The listing builds one solid part. Answer for the finished solid, in the listing's coordinates (mm). A direction names the side the tool comes from. Give positions to 0.01 mm unless a question says otherwise; leave off trailing zeros. Loops run counter-clockwise (first coordinate to the right, second up) from the corner with the lowest first, then second, coordinate; pieces in that order, holes last. Notation, with made-up numbers: M 13,-16 L 23,-16 A11 ccw 23,-11 Z; hole C -5,24.25 d10. An arc over 180 degrees is marked long. One line per item, written item: value. Start each with the question number.
Q1. A cutting plane is placed at C-C, the plane z = -20.3. Determine the outline of the cut face in (x, y), and give its area (3 significant figures).
Q2. A cutting plane is placed at B-B, the plane x = 1.65. Determine the outline of the cut face in (y, z), and give its area (3 significant figures).
Q3. The mould has two halves that part along Y. Classify faces 3 (the cylindrical face through (-0.04, 8.54, -41.03)), 4 (the cylindrical face through (1, 9, -48)), 5 (the cylindrical face through (0.035, -3.212, -2.502)): +Y half, -Y half, draft (parallel to the pull), parting line (faces both ways), or undercut.
Q4. A cutting plane is placed at D-D, the plane z = -39.5. Determine the outline of the cut face in (x, y).
Q5. Consider L1, parallel to Y at x = -0.15, z = -20.3; L2, parallel to Y at x = -1.9, z = -29.5; L3, parallel to Y at x = -1.4, z = -40. Determine where each line is inside the solid, lowest interval first.
Q6. Flat-ended cylindrical pins translate along their axes: pin 1 (1.5 mm diameter, centred on x = 1, z = -28, fed in from +Y); pin 2 (3 mm diameter, centred on x = 1, y = -8, fed in from +Z). Find the tip coordinate at first contact, or state that the pin passes through.
Q7. For faces 1 (the flat face through (-2.5, -1, -25)), 2 (the flat face through (1, 10, -53)), determine the directions among +Z, -Z, +X, -X, +Y, -Y from which every point of the face is accessible in a straight line to the end or side of a thin tool.
Q8. A cutting plane is placed at A-A, the plane y = -10.8. Determine the outline of the cut face in (x, z), and give its area (3 significant figures).
from build123d import *

# Parameters (mm, degrees)
ESQUISSE1_W             = 5
ESQUISSE1_H             = 28
EXTRUSION1_DEPTH        = 46
ESQUISSE2_R             = 2
ESQUISSE2_R_2           = 3.5
EXTRUSION2_DEPTH        = 49.342527861
TROU_TARAUD_M21_D       = 1.6
BOSS_EXTRU_2_DEPTH      = 5
ENL_V_MAT_EXTRU_1_DEPTH = 10
ENL_V_START             = 3
ENL_V_MAT_EXTRU_2_DEPTH = 56.9067059


with BuildPart() as part:
    # Esquisse1 → Extrusion1 (new body)
    with BuildSketch(Plane.XY):
        Rectangle(ESQUISSE1_W, ESQUISSE1_H)
    extrude(amount=-EXTRUSION1_DEPTH)

    # Esquisse2 → Extrusion2 (cut, through all)
    with BuildSketch(Plane(origin=(2.5, 0, 0), x_dir=(0, 0, -1), z_dir=(1, 0, 0))):
        with Locations((4.5, -3.3)):
            Circle(ESQUISSE2_R)
        with Locations((40, -3.3)):
            Circle(ESQUISSE2_R_2)
    extrude(amount=-EXTRUSION2_DEPTH, mode=Mode.SUBTRACT)

    # Trou taraudé M21 (through all)
    with Locations(Plane(origin=(2.5, 0, 0), x_dir=(0, 0, -1), z_dir=(1, 0, 0))):
        with Locations((20.3, 4.2), (20.3, -10.8)):
            Hole(TROU_TARAUD_M21_D / 2)

    # Esquisse12 → Boss.-Extru.2 (add)
    with BuildSketch(Plane.ZY.offset(2.5)):
        with BuildLine():
            Line((-46, 14), (-50.208712153, 14))
            ThreePointArc((-50.208712153, 14), (-52.5, 12.5), (-54.791287847, 14))
            Line((-54.791287847, 14), (-55, 14))
            ThreePointArc((-55, 14), (-57, 12), (-55, 10))
            Line((-55, 10), (-50, 10))
            ThreePointArc((-50, 10), (-48.294604063, 9.328011132), (-47.506013794, 7.673299759))
            Line((-47.506013794, 7.673299759), (-46, -14))
            Line((-46, -14), (-46, 14))
        make_face()
    extrude(amount=-BOSS_EXTRU_2_DEPTH)

    # Esquisse13 → Enlèv. mat.-Extru.1 (cut)
    with BuildSketch(Plane.ZY.offset(2.5)):
        with BuildLine():
            ThreePointArc((-47.521517479, 7.82729863), (-47.512573575, 7.750419205), (-47.506013794, 7.673299759))
            Line((-47.506013794, 7.673299759), (-46, -14))
            Line((-46, -14), (-36, -14))
            ThreePointArc((-36, -14), (-37.164860583, -13.780452956), (-38.169882605, -13.151937389))
            Line((-38.169882605, -13.151937389), (-44.068529884, -7.709882605))
            ThreePointArc((-44.068529884, -7.709882605), (-45.326210473, -6.062513711), (-45.94835805, -4.085516713))
            Line((-45.94835805, -4.085516713), (-47.521517479, 7.82729863))
        make_face()
        with BuildLine():
            ThreePointArc((-18.401732057, -13.767179458), (-18.989661678, -13.941255662), (-19.6, -14))
            Line((-19.6, -14), (0, -14))
            Line((0, -14), (0, -3.3))
            ThreePointArc((0, -3.3), (-0.769531576, -5.81666552), (-2.814935705, -7.472596113))
            Line((-2.814935705, -7.472596113), (-18.401732057, -13.767179458))
        make_face()
        with BuildLine():
            ThreePointArc((-2.814935705, 0.872596113), (-0.769531576, -0.78333448), (0, -3.3))
            Line((0, -3.3), (0, 14))
            Line((0, 14), (-50, 14))
            ThreePointArc((-50, 14), (-47.228274994, 13.379416679), (-44.985807313, 11.636166305))
            ThreePointArc((-44.985807313, 11.636166305), (-40.96713796, 8.512131601), (-36, 7.4))
            Line((-36, 7.4), (-19.6, 7.4))
            ThreePointArc((-19.6, 7.4), (-18.989661678, 7.341255662), (-18.401732057, 7.167179458))
            Line((-18.401732057, 7.167179458), (-2.814935705, 0.872596113))
        make_face()
    extrude(amount=-ENL_V_MAT_EXTRU_1_DEPTH, mode=Mode.SUBTRACT)

    # Esquisse14 → Enlèv. mat.-Extru.2 (cut, through all)
    with BuildSketch(Plane.ZY.offset(-2.5).offset(ENL_V_START)):
        with BuildLine():
            ThreePointArc((-44.985807313, 11.636166305), (-47.228274994, 13.379416679), (-50, 14))
            Line((-50, 14), (-50.208712153, 14))
            ThreePointArc((-50.208712153, 14), (-52.5, 12.5), (-54.791287847, 14))
            Line((-54.791287847, 14), (-55, 14))
            ThreePointArc((-55, 14), (-57, 12), (-55, 10))
            Line((-55, 10), (-50, 10))
            ThreePointArc((-50, 10), (-48.933951921, 9.761314107), (-48.071464351, 9.090833194))
            ThreePointArc((-48.071464351, 9.090833194), (-47.801302388, 11.906328268), (-44.985807313, 11.636166305))
        make_face()
    extrude(amount=ENL_V_MAT_EXTRU_2_DEPTH, mode=Mode.SUBTRACT)


solid = part.part
Answer block:
1. outline: M -2.5,-14 L 2.5,-14 L 2.5,-11.6 L -2.5,-11.6 Z; M -2.5,-10 L 2.5,-10 L 2.5,3.4 L -2.5,3.4 Z; M -2.5,5 L 2.5,5 L 2.5,7.4 L -2.5,7.4 Z
1. area: 91.0 mm^2
2. outline: M -14,-36 A3.2 ccw -13.15,-38.17 L -7.71,-44.07 A6 ccw -4.09,-45.95 L 7.83,-47.52 A2.5 cw 10,-50 L 10,-55 A2 ccw 14,-55 L 14,-54.79 A2.5 cw 14,-50.21 L 14,-50 A6.5 ccw 11.64,-44.99 A11.65 cw 7.4,-36 L 7.4,-19.6 A3.2 ccw 7.17,-18.4 L 0.87,-2.81 A4.5 ccw -7.47,-2.81 L -13.77,-18.4 A3.2 ccw -14,-19.6 Z; hole C -10.8,-20.3 d1.6; hole C -3.3,-40 d7; hole C -3.3,-4.5 d4; hole C 4.2,-20.3 d1.6
2. area: 810 mm^2
3. face 3: +Y half
3. face 4: -Y half
3. face 5: undercut
4. outline: M -2.5,-11.92 L 2.5,-11.92 L 2.5,-6.76 L -2.5,-6.76 Z; M -2.5,0.16 L 2.5,0.16 L 2.5,7.94 L -2.5,7.94 Z
5. L1: -14 to -11.6, -10 to 3.4, 5 to 7.4
5. L2: -14 to 7.4
5. L3: -11.46 to -6.8, 0.2 to 8.11
6. pin 1: y = 7.4
6. pin 2: z = -1.34
7. face 1: +Z, -Z, -X, +Y, -Y
7. face 2: -Z, +X, -X, -Y
8. outline: M -2.5,-40.72 L 2.5,-40.72 L 2.5,-21.1 L -2.5,-21.1 Z; M -2.5,-19.5 L 2.5,-19.5 L 2.5,-11.05 L -2.5,-11.05 Z
8. area: 140 mm^2
